from build123d import *

# Parameters (mm, degrees)
SZKIC1_R                    = 6.5
DODANIE_WYCI_GNI_CIE3_DEPTH = 5
SFAZOWANIE3_SIZE            = 0.5


with BuildPart() as part:
    # Szkic1 → Dodanie-wyciągnięcie3 (new body)
    with BuildSketch(Plane.XY):
        Polygon((9.237604307, 0), (4.618802154, 8), (-4.618802154, 8), (-9.237604307, 0), (-4.618802154, -8), (4.618802154, -8), align=None)
        Circle(SZKIC1_R, mode=Mode.SUBTRACT)
    extrude(amount=DODANIE_WYCI_GNI_CIE3_DEPTH)

    # Szkic2 → Wycięcie-obrót3 (revolve, cut)
    with BuildSketch(Plane(origin=(0, 0, 0), x_dir=(1, 0, 0), z_dir=(0, 1, 0))):
        Polygon((9.237604307, -5), (9.237604307, -4), (8.237604307, -5), align=None)
    revolve(axis=Axis((0, 0, 0), (0, 0, 1)), mode=Mode.SUBTRACT)

    # Sfazowanie3
    sfazowanie3_edges = [part.edges().sort_by_distance(p)[0] for p in [
        (-6.5, 0, 0),
    ]]
    chamfer(sfazowanie3_edges, length=SFAZOWANIE3_SIZE)


solid = part.part
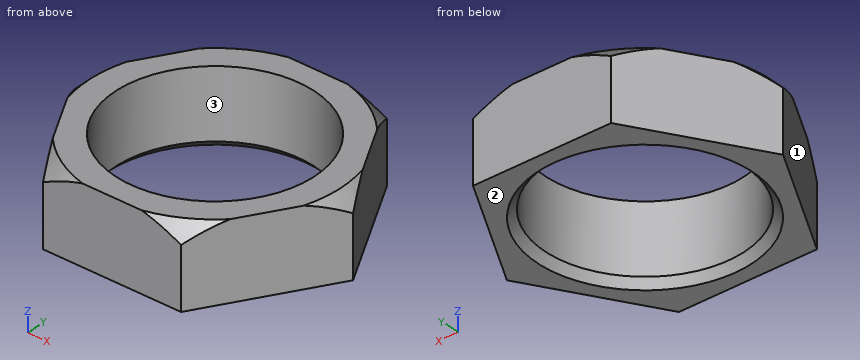
Part model, mm, in its own coordinate system. Face numbers are marked on the shaded views. Coordinates: 2 decimals unless noted, no trailing zeros. Loops run counter-clockwise (first coordinate to the right, second up) from the corner with the lowest first, then second, coordinate; pieces in that order, holes last. Notation, with made-up numbers: (-32.5, 17.25) -> (7.5, 17.25) arc R10 cw to (7.5, 33.25) -> close; hole circle Ø5 at (-4, -5.5). An arc over 180 degrees is marked (long way). Use a Markdown table: item, result. Add a question column.
Item 1: Band-saw the part on C-C on z = 4.5. Write the cut outline in (x, y).
Item 2: Pull direction X, two halves, no side cores. Call the marked faces 1, 2 and 3: +X half, -X half, draft (parallel to the pull), parting line (faces both ways), or undercut.
Item 3: Band-saw the part on B-B on z = 1.9. Write the cut outline in (x, y).
Item 4: Probe probe 1 along Y at (x, z) = (0, 4.15); probe 2 along X at (y, z) = (5.25, 4.2); probe 3 along X at (y, z) = (-0.25, 2.6). List the from-to ranges inside material, lowest first.
Item 5: Band-saw the part on A-A on x = 0. Write the cut outline in (y, z).
Item 6: Flat gauge pins, fed straight in: P1, Ø5, axis at x = -7, y = -4.5, coming from the +Z side; P2, Ø3, axis at y = 2.5, z = 3.5, coming from the +X side. Where does each tip first touch, or does it go through?
Geometry says:
| question | item | result |
|---|---|---|
| 1 | outline | (-8.69, -0.96) -> (-5.17, -7.04) arc R8.74 ccw to (-3.51, -8) -> (3.51, -8) arc R8.74 ccw to (5.17, -7.04) -> (8.69, -0.96) arc R8.74 ccw to (8.69, 0.96) -> (5.17, 7.04) arc R8.74 ccw to (3.51, 8) -> (-3.51, 8) arc R8.74 ccw to (-5.17, 7.04) -> (-8.69, 0.96) arc R8.74 ccw to start; hole circle Ø13 at (0, 0) |
| 2 | face 1 | -X half |
| 2 | face 2 | draft |
| 2 | face 3 | undercut |
| 3 | outline | (-9.24, 0) -> (-4.62, -8) -> (4.62, -8) -> (9.24, 0) -> (4.62, 8) -> (-4.62, 8) -> close; hole circle Ø13 at (0, 0) |
| 4 | probe 1 | -8 to -6.5, 6.5 to 8 |
| 4 | probe 2 | -6.21 to -3.83, 3.83 to 6.21 |
| 4 | probe 3 | -9.09 to -6.5, 6.5 to 9.09 |
| 5 | outline | (-8, 0) -> (-7, 0) -> (-6.5, 0.5) -> (-6.5, 5) -> (-8, 5) -> close; (6.5, 0.5) -> (7, 0) -> (8, 0) -> (8, 5) -> (6.5, 5) -> close |
| 6 | P1 | z = 5 |
| 6 | P2 | x = 8.66 |
